Build history of the part. All positions in model axes, mm. Coordinates: 2 decimals unless noted, no trailing zeros. Loops run counter-clockwise (first coordinate to the right, second up) from the corner with the lowest first, then second, coordinate; pieces in that order, holes last.
(1) Slice it at A-A (x = 51.5). Give the cut face in (y, z), and give its area (3 significant figures).
(2) Slice it at C-C (z = 0.4). Give the number of separate pieces and of enclosed holes in the cut face, and give its area (3 significant figures).
(3) Wall check: L1, parallel to Y at x = 75, z = 0.9; L2, parallel to Y at x = -44, z = 0.4; L3, parallel to Y at x = 82.5, z = 0.4. Give the ranges that are in metal, low to high.
(4) Slice it at B-B (x = -4). Give the cut face in (y, z), and give its area (3 significant figures).
(5) Flat gauge pins, fed straight in: P1, Ø6.5, axis at x = 51.5, y = 22, coming from the -Z side; P2, Ø8, axis at x = -54, y = 22, coming from the +Z side. Where does each tip first touch, or does it go through?
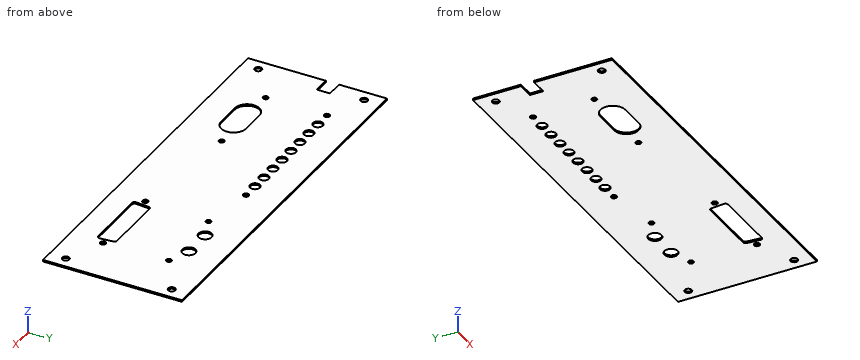
from build123d import *

# Parameters (mm, degrees)
SKETCH_1_W          = 228
SKETCH_1_H          = 84
SKETCH_1_R          = 2.15
EXTRUDE_1_DEPTH     = 1
SKETCH_3_R          = 1.7
SKETCH_3_R_2        = 1.6
SKETCH_3_R_3        = 4
CUT_EXTRUDE_1_DEPTH = 10
SKETCH_4_R          = 1.6
SKETCH_4_W          = 16.398551469
SKETCH_4_H          = 8
CUT_EXTRUDE_2_DEPTH = 1
SKETCH_5_R          = 1.7
SKETCH_5_R_2        = 3
CUT_EXTRUDE_3_DEPTH = 10


with BuildPart() as part:
    # Эскиз1 → Вытянуть1 (new body)
    with BuildSketch(Plane.XY):
        Rectangle(SKETCH_1_W, SKETCH_1_H)
        with Locations((107, 32)):
            Circle(SKETCH_1_R, mode=Mode.SUBTRACT)
        with Locations(Location((-107, 32, 0), (0, 0, 180))):
            Circle(SKETCH_1_R, mode=Mode.SUBTRACT)
        with Locations((-107, -32)):
            Circle(SKETCH_1_R, mode=Mode.SUBTRACT)
        with Locations(Location((107, -32, 0), (0, 0, 180))):
            Circle(SKETCH_1_R, mode=Mode.SUBTRACT)
    extrude(amount=EXTRUDE_1_DEPTH)

    # Эскиз3 → Вырез-Вытянуть1 (cut)
    with BuildSketch(Plane.XY.offset(1)):
        with Locations((37, -22)):
            Circle(SKETCH_3_R)
        with Locations((84, -22)):
            Circle(SKETCH_3_R)
        with Locations((38.5, 17)):
            Circle(SKETCH_3_R_2)
        with Locations((82.5, 17)):
            Circle(SKETCH_3_R_2)
        with Locations((51.5, 22)):
            Circle(SKETCH_3_R_3)
        with Locations((69.5, 22)):
            Circle(SKETCH_3_R_3)
        with BuildLine():
            Line((40.14870942, -25.864196381), (40.875982147, -17.864196381))
            ThreePointArc((40.875982147, -17.864196381), (41.358314525, -16.892366164), (42.369821957, -16.5))
            Line((42.369821957, -16.5), (78.630178043, -16.5))
            ThreePointArc((78.630178043, -16.5), (79.641685475, -16.892366164), (80.124017853, -17.864196381))
            Line((80.124017853, -17.864196381), (80.85129058, -25.864196381))
            ThreePointArc((80.85129058, -25.864196381), (80.465084606, -27.011507432), (79.35745077, -27.5))
            Line((79.35745077, -27.5), (41.64254923, -27.5))
            ThreePointArc((41.64254923, -27.5), (40.534915394, -27.011507432), (40.14870942, -25.864196381))
        make_face()
    extrude(amount=-CUT_EXTRUDE_1_DEPTH, mode=Mode.SUBTRACT)

    # Эскиз4 → Вырез-Вытянуть2 (cut)
    with BuildSketch(Plane.XY.offset(1)):
        with Locations((-84, -15)):
            Circle(SKETCH_4_R)
        with Locations((-35, -15)):
            Circle(SKETCH_4_R)
        with BuildLine():
            Line((-67, -9.5), (-52, -9.5))
            ThreePointArc((-52, -9.5), (-44.5, -17), (-52, -24.5))
            Line((-52, -24.5), (-67, -24.5))
            ThreePointArc((-67, -24.5), (-74.5, -17), (-67, -9.5))
        make_face()
        with Locations((-112.199275735, 9)):
            Rectangle(SKETCH_4_W, SKETCH_4_H)
    extrude(amount=-CUT_EXTRUDE_2_DEPTH, mode=Mode.SUBTRACT)

    # Эскиз5 → Вырез-Вытянуть3 (cut)
    with BuildSketch(Plane.XY.offset(1)):
        with Locations((-84, 22)):
            Circle(SKETCH_5_R)
        with Locations((6, 22)):
            Circle(SKETCH_5_R)
        with Locations((-4, 22)):
            Circle(SKETCH_5_R_2)
        with Locations((-14, 22)):
            Circle(SKETCH_5_R_2)
        with Locations((-24, 22)):
            Circle(SKETCH_5_R_2)
        with Locations((-34, 22)):
            Circle(SKETCH_5_R_2)
        with Locations((-44, 22)):
            Circle(SKETCH_5_R_2)
        with Locations((-54, 22)):
            Circle(SKETCH_5_R_2)
        with Locations((-64, 22)):
            Circle(SKETCH_5_R_2)
        with Locations((-74, 22)):
            Circle(SKETCH_5_R_2)
    extrude(amount=-CUT_EXTRUDE_3_DEPTH, mode=Mode.SUBTRACT)


solid = part.part
Response values:
1. outline: (-42, 0) - (-27.5, 0) - (-27.5, 1) - (-42, 1) - close; (-16.5, 0) - (18, 0) - (18, 1) - (-16.5, 1) - close; (26, 0) - (42, 0) - (42, 1) - (26, 1) - close
1. area: 65.0 mm2
2. separate pieces: 1
2. enclosed holes: 24
2. area: 17,800 mm2
3. L1: y = -42 to -27.5, -16.5 to 42
3. L2: y = -42 to 19, 25 to 42
3. L3: y = -42 to -22.8, -21.2 to 15.4, 18.6 to 42
4. outline: (-42, 0) - (19, 0) - (19, 1) - (-42, 1) - close; (25, 0) - (42, 0) - (42, 1) - (25, 1) - close
4. area: 78.0 mm2
5. P1: passes through
5. P2: stops at z = 1
